For this review, take the finished solid that the model builds, in its own axes (mm). A direction names the side the tool comes from. Round coordinates to 2 decimals unless told otherwise and drop trailing zeros. Write each loop counter-clockwise with the first axis right and the second up, starting at its lowest first coordinate (ties: lowest second). Pieces come first, ordered by that corner, then holes.
Autodesk Inventor part; units mm, degrees
ref_plane "РабПлоскость1" through (0, 0, 8.25) normal (0, 0, 1) x (1, 0, 0)
sketch "Эскиз1" plane through (0, 0, 8.25) normal (0, 0, 1) x (1, 0, 0)
  circle A0 centre (0, 0) radius 17.5
  circle A1 centre (0, 0) radius 6
  dimension "d1" = 35
  dimension "d2" = 12
extrude "Выдавливание1" add sketch "Эскиз1" along normal blind 43
ref_plane "РабПлоскость2" through (0, -17.5, 8.25) normal (0, 1, 0) x (-1, 0, 0)
ref_plane "РабПлоскость3" through (-17.5, 0, 8.25) normal (1, 0, 0) x (0, 1, 0)
sketch "Эскиз2" plane through (-17.5, 0, 8.25) normal (1, 0, 0) x (0, 1, 0)
  line L0 (17.5, 43) -> (-17.5, 43)
  line L1 (0, 43) -> (0, 0) construction
  line L2 (17.5, 0) -> (-17.5, 0)
  circle A0 centre (0, 21.5) radius 13
  point P0 (0, -8.25)
  dimension "d23" = 26
extrude "Выдавливание2" add sketch "Эскиз2" along normal up to surface
sketch "Эскиз3" plane through (-17.5, 0, 8.25) normal (-1, 0, 0) x (0, 0, 1)
  arc A0 (8.5, 0) -> (34.5, 0) centre (21.5, 0) ccw construction
  circle A1 centre (21.5, 0) radius 13
  point P0 (-8.25, 0)
  point P1 (40, 0)
  point P2 (5, 0)
  point P3 (39, 0)
  point P4 (4, 0)
  point P5 (6.5, 0)
  point P6 (36.5, 0)
extrude "Выдавливание3" add sketch "Эскиз3" along normal blind 6
fillet "Сопряжение1" radius 5 3 edges at (-11.7154, -13, 29.7735) (-14.4476, 9.875, 21.2952) (-14.4454, 9.8782, 38.201)
fillet "Сопряжение2" radius 2 2 edges at (-17.5, 0, 8.25) (-17.5, 0, 51.25)
sketch "Эскиз5" plane through (-23.5, 0, 29.75) normal (-1, 0, 0) x (0, 0, 1)
  circle A0 centre (0, 0) radius 5
  circle A1 centre (0, 0) radius 10 construction
  circle A2 centre (0, 10) radius 2.2
  circle A3 centre (-7.8183, 6.2349) radius 2.2
  circle A4 centre (-9.7493, -2.2252) radius 2.2
  circle A5 centre (-4.3388, -9.0097) radius 2.2
  circle A6 centre (4.3388, -9.0097) radius 2.2
  circle A7 centre (9.7493, -2.2252) radius 2.2
  circle A8 centre (7.8183, 6.2349) radius 2.2
  point P0 (-29.75, 0)
  dimension "d17" = 20
  dimension "d14" = 10
  dimension "d18" = 4.4
  dimension "d21" = 360
extrude "Выдавливание5" cut sketch "Эскиз5" against normal blind 15.5
sketch "Эскиз6" plane through (0, 0, 8.25) normal (0, 0, -1) x (-1, 0, 0)
  line L0 (-2.1, 2.2009) -> (2.1, 2.2009)
  line L1 (2.1, 2.2009) -> (2.1, 7.8)
  line L2 (2.1, 7.8) -> (-2.1, 7.8)
  line L3 (-2.1, 7.8) -> (-2.1, 2.2009)
  line L4 (-2.1, 2.2009) -> (2.1, 7.8) construction
  line L5 (2.1, 2.2009) -> (-2.1, 7.8) construction
  circle A0 centre (0, 0) radius 6
  point P0 (0, 5.0005)
  point P1 (-2.1, 5.6205)
  point P2 (2.1, 5.6205)
  dimension "d24" = 4.2
  dimension "d25" = 7.8
extrude "Выдавливание6" cut sketch "Эскиз6" against normal through all contours L3 L2 L1 A0
sketch "Эскиз7" plane through (0, 0, 51.25) normal (0, 0, 1) x (1, 0, 0)
  arc A0 (-2.1, 5.6205) -> (2.1, 5.6205) centre (0, 0) ccw construction
  line L0 (2.1, 7.8) -> (2.1, 5.6205) construction
  line L1 (-2.1, 5.6205) -> (-2.1, 7.8) construction
  line L2 (-2.1, 7.8) -> (2.1, 7.8) construction
  arc A1 (-2.2, 5.6895) -> (2.2, 5.6895) centre (0, 0) ccw
  line L3 (-2.2, 5.6895) -> (-2.2, 7.9)
  line L4 (-2.2, 7.9) -> (2.2, 7.9)
  line L5 (2.2, 7.9) -> (2.2, 5.6895)
  dimension "d28" = 0.1
extrude "Выдавливание7" cut sketch "Эскиз7" against normal blind 56.75
properties part number "Крпеление ОУ"
(1) We need section A-A, the plane x = 0. Give the boundary of the cut face in (y, z).
Geometry check:
outline: (-17.5, 10.25) arc R2 ccw to (-15.5, 8.25) - (-6.1, 8.25) - (-6.1, 51.25) - (-15.5, 51.25) arc R2 ccw to (-17.5, 49.25) - close; (7.9, 8.25) - (15.5, 8.25) arc R2 ccw to (17.5, 10.25) - (17.5, 49.25) arc R2 ccw to (15.5, 51.25) - (7.9, 51.25) - close
(2) Mouldability with a two-part tool opening along Y and no side actions: class faces 1 (the face through (16.166, 6.703, 29.477)), 2 (the face through (-15.858, 0.22, 24.755)), 3 (the face through (-8, -2, 39)), 4 (the face through (0, -7, 51.25)) as pulls with the +Y half, pulls with the -Y half, needs draft (parallel to the pull), parting line crosses it, or undercut.
Geometry check:
face 1: parting line crosses it
face 2: undercut
face 3: undercut
face 4: needs draft
(3) For faces 5 (the face through (-23.5, 0, 35)), 6 (the face through (-15.86, -0.37, 21.18)), 7 (the face through (2.2, 7, 30)), list the 3-axis set-ups (+Z, -Z, +X, -X, +Y, -Y) from which the entire face can be reached by the end or side of a thin tool; tool diameter is ignored.
Geometry check:
face 5: +Z, -Z, -X, +Y, -Y
face 6: -X
face 7: +Z, -Z
(4) For pin 1 Ø7 at (y, z) = (6.23, 37.57) entering from -X; pin 2 Ø4 at (x, z) = (13, 27.5) entering from -Y; pin 3 Ø3.5 at (y, z) = (-9.01, 34.09) entering from +X; pin 4 Ø2.5 at (y, z) = (10, 29.75) entering from +X, all flat-tipped, find the tip position at first contact; note any pin that passes through.
Geometry check:
pin 1: stops at x = -23.5
pin 2: stops at y = -13.61
pin 3: stops at x = 15.92
pin 4: stops at x = 15.16
(5) For line 1 along Y through (x, z) = (-13.25, 29.75); line 2 along Y through (x, z) = (-11.5, 26.5); line 3 along X through (y, z) = (-5, 22), list the stretches that pass through material, from the lowest coordinate up.
Geometry check:
line 1: y = -13.01 to -5, 5 to 7.8, 12.2 to 13.01
line 2: y = -13.3 to -10.92, -7.1 to -3.8, 3.8 to 13.3
line 3: x = -23.5 to -3.49, 3.49 to 16.77
